```python
from build123d import *

# Parameters (mm, degrees)
SKETCH1_W                       = 22.225
SKETCH1_H                       = 5.588
REVOLVE1_ANGLE                  = 27
SKETCH2_R                       = 2.049999964
SKETCH2_W                       = 6.99999997
SKETCH2_H                       = 10.000000066
CUT_EXTRUDE1_DEPTH              = 8.468834779
FILLET2_R                       = 2.54
BOSS_EXTRUDE2_DEPTH             = 25.4
BOSS_EXTRUDE2_DEPTH_BACK        = 1.27
F_24_0_152_DIAMETER_HOLE1_D     = 3.8608
F_24_0_152_DIAMETER_HOLE1_DEPTH = 3.3999932
F_24_0_152_DIAMETER_HOLE1_TIP   = 1.159901339


with BuildPart() as part:
    # Sketch1 → Revolve1 (revolve, symmetric)
    with BuildSketch(Plane.XY) as revolve1_sk:
        with Locations((0, -2.794)):
            Rectangle(SKETCH1_W, SKETCH1_H)
    revolve(axis=Axis((21.580970856, -73.66, 0), (-1, 0, 0)), revolution_arc=REVOLVE1_ANGLE / 2)
    revolve(revolve1_sk.sketch, axis=Axis((21.580970856, -73.66, 0), (1, 0, 0)), revolution_arc=REVOLVE1_ANGLE / 2)

    # Sketch2 → Cut-Extrude1 (cut, through all)
    with BuildSketch(Plane(origin=(0, 0, 0), x_dir=(1, 0, 0), z_dir=(0, 1, 0))):
        with Locations((-5.231250015, 12.7)):
            Circle(SKETCH2_R)
        with Locations((-5.231250015, -12.7)):
            Circle(SKETCH2_R)
        with Locations((-5.231250015, 0)):
            Rectangle(SKETCH2_W, SKETCH2_H)
    extrude(amount=-CUT_EXTRUDE1_DEPTH, mode=Mode.SUBTRACT)

    # Fillet2
    fillet2_edges = [part.edges().sort_by_distance(p)[0] for p in [
        (-11.1125, -4.752033221, 16.543339155),
        (-11.1125, -4.752033221, -16.543339155),
    ]]
    fillet(fillet2_edges, radius=FILLET2_R)

    # Sketch8 → Boss-Extrude2 (add, two sides)
    with BuildSketch(Plane(origin=(11.1125, 0, 0), x_dir=(0, 0, -1), z_dir=(1, 0, 0))) as boss_extrude2_sk:
        with BuildLine():
            Line((-15, -7.874), (15, -7.874))
            Line((15, -7.874), (15.184616566, -1.5821045))
            ThreePointArc((15.184616566, -1.5821045), (0.094309083, -6.0373e-05), (-15, -1.543458208))
            Line((-15, -1.543458208), (-15, -7.874))
        make_face()
    extrude(amount=BOSS_EXTRUDE2_DEPTH)
    extrude(boss_extrude2_sk.sketch, amount=-BOSS_EXTRUDE2_DEPTH_BACK)

    # 24 _0.152_ Diameter Hole1
    with Locations(Plane(origin=(0, -7.874, 0), x_dir=(-1, 0, 0), z_dir=(0, -1, 0))):
        with Locations((-32.26874997, 11.5), (-32.26874997, -11.5)):
            Hole(F_24_0_152_DIAMETER_HOLE1_D / 2, depth=F_24_0_152_DIAMETER_HOLE1_DEPTH)
            with Locations((0, 0, -(F_24_0_152_DIAMETER_HOLE1_DEPTH + F_24_0_152_DIAMETER_HOLE1_TIP / 2))):  # 118° drill point
                Cone(0, F_24_0_152_DIAMETER_HOLE1_D / 2, F_24_0_152_DIAMETER_HOLE1_TIP, mode=Mode.SUBTRACT)


solid = part.part
```
Here's how the part is built. I have some questions about the finished solid (model axes, mm). A direction names the side the tool comes from. Round coordinates to 2 decimals unless told otherwise and drop trailing zeros. Order: outer loops, then holes, each group sorted by start corner. A loop starts at its lowest first (then second) coordinate and runs counter-clockwise, first axis right, second up. Notation, with made-up numbers: M 59,-18 L 80,-18 A22 cw 80,-11 Z; hole C -10,30 d7. An arc over 180 degrees is marked long. Answer as CSV lines item,"result".
Item 1: We'd pull the mould along Z, two halves only. Please class faces 5 (the flat face through (-11.113, -3, 0)), 6 (the cylindrical face through (-10.39, -4.56, 15.8)), 7 (the cylindrical face through (0.16, -5.59, -0.22)): +Z half, -Z half, draft (parallel to the pull), parting line (faces both ways), or undercut.
From the geometry:
face 5,"draft"
face 6,"+Z half"
face 7,"undercut"
Item 2: Imagine slicing it at B-B on z = -6. List the corners of the cut face in (x, y) for me, and give its area (3 significant figures).
From the geometry:
outline,"M -11.11,-5.85 L 9.84,-5.85 L 9.84,-7.87 L 36.51,-7.87 L 36.51,-0.24 L -11.11,-0.24 Z"
area,"321 mm2"
Item 3: Which directions (+Z, -Z, +X, -X, +Y, -Y) give clear straight access to the entire face, cutting with the end or side of a thin tool? Please do faces 1 (the flat face through (9.843, -7, 0)), 2 (the cylindrical face through (34.05, -6.15, -10.76)), 3 (the flat face through (-1.731, -3, 0)), 4 (the flat face through (11.112, -4, 16)).
From the geometry:
face 1,"-X, -Y"
face 2,"-Y"
face 3,"+Y, -Y"
face 4,"+Z, +X, +Y, -Y"
Item 4: Please list where these lines run through material, in increasing order: L1, parallel to X at y = -4, z = -12.7; L2, parallel to X at y = -2, z = -3; L3, parallel to X at y = -6.1, z = -11.5. Write a range as [from, to].
From the geometry:
L1,"[-11.11, -7.28], [-3.18, 36.51]"
L2,"[-11.11, -8.73], [-1.73, 36.51]"
L3,"[-11.11, -6.89], [-3.57, 30.34], [34.2, 36.51]"
Item 5: For pin 1 (4.5 mm diameter, centred on x = 32.27, z = 11.5, fed in from +Y); pin 2 (5.5 mm diameter, centred on x = -5.23, z = 12.7, fed in from -Y); pin 3 (2 mm diameter, centred on x = 13.5, z = -7, fed in from +Y), each with a flat end and sliding along its axis, tell me the tip position at first contact or that it passes through.
From the geometry:
pin 1,"y = -0.58"
pin 2,"y = -7.36"
pin 3,"y = -0.24"
Item 6: Imagine slicing it at A-A on x = 2. List the corners of the cut face in (y, z) for me, and give its area (3 significant figures).
From the geometry:
outline,"M -7.47,-15.89 L -2.04,-17.2 A73.66 ccw -2.04,17.2 L -7.47,15.89 A68.07 cw Z"
area,"187 mm2"
